Design review of the part built by this model. Coordinates are the model's own, in mm. A direction names the side the tool comes from. Coordinates: 2 decimals unless noted, no trailing zeros. Loops run counter-clockwise (first coordinate to the right, second up) from the corner with the lowest first, then second, coordinate; pieces in that order, holes last. Notation, with made-up numbers: (-2.75, -34.75) -> (17.25, -34.75) arc R9 ccw to (17.25, -18.75) -> close; hole circle Ø8 at (55.5, 66.25). An arc over 180 degrees is marked (long way). Use a Markdown table: item, result. Add a question column.
Q1. For faces 4 (the face through (-14.287, 14.248, 2.028)), 5 (the face through (11, -8, 11)), list the 3-axis set-ups (+Z, -Z, +X, -X, +Y, -Y) from which the entire face can be reached by the end or side of a thin tool; tool diameter is ignored.
Q2. For probe 1 along Y at (x, z) = (0, 1.2); probe 2 along X at (y, z) = (-5.5, 5); probe 3 along Z at (x, y) = (-6, 1.5), list the stretches that pass through material, from the lowest coordinate up.
Q3. Clearance check with flat-ended pins moving along their axes: pin 1 Ø6 at (x, y) = (-4, 0.5) entering from -Z; pin 2 Ø6 at (x, y) = (6, 6) entering from +Z; pin 3 Ø7.5 at (x, y) = (0, 0) entering from +Z. State where each tip first meets the part, or that it passes through.
Q4. Take a section at A-A on z = 29. Write out the cut boundary in (x, y), plus the area to 3 significant figures.
Q5. Draft analysis for pull direction X (two halves, no side actions). For faces 1 (the face through (0, 15, 2)), 2 (the face through (-15, -5, 12)), 3 (the face through (-11, -8, 11)), state which applies: pulls with the +X half, pulls with the -X half, needs draft (parallel to the pull), parting line crosses it, or undercut.
Q6. Take a section at D-D on y = -9. Write out the cut boundary in (x, z), plus the area to 3 significant figures.
Q7. Take a section at C-C on x = 0. Write out the cut boundary in (y, z), plus the area to 3 significant figures.
Q8. Take a section at B-B on y = 0. Write out the cut boundary in (x, z), plus the area to 3 significant figures.
from build123d import *

# Parameters (mm, degrees)
ESQUISSE1_W             = 30
ESQUISSE1_H             = 33
ESQUISSE1_R             = 4.25
BOSS_EXTRU_1_DEPTH      = 4
CONG_1_R                = 2.5
BOSS_EXTRU_2_DEPTH      = 4
BOSS_EXTRU_3_DEPTH      = 4
ESQUISSE5_R             = 150
ENL_V_MAT_EXTRU_1_DEPTH = 42.291645644


with BuildPart() as part:
    # Esquisse1 → Boss.-Extru.1 (new body)
    with BuildSketch(Plane.XY):
        with Locations((0, -1.5)):
            Rectangle(ESQUISSE1_W, ESQUISSE1_H)
        Circle(ESQUISSE1_R, mode=Mode.SUBTRACT)
    extrude(amount=BOSS_EXTRU_1_DEPTH)

    # Congé1
    cong_1_edges = [part.edges().sort_by_distance(p)[0] for p in [
        (-15, 15, 2),
        (15, 15, 2),
    ]]
    fillet(cong_1_edges, radius=CONG_1_R)

    # Esquisse2 → Boss.-Extru.2 (add)
    with BuildSketch(Plane(origin=(15, 0, 0), x_dir=(0, 0, -1), z_dir=(1, 0, 0))):
        Polygon((-4, -18), (-34, -18), (-4, 12), align=None)
    extrude(amount=-BOSS_EXTRU_2_DEPTH)

    # Esquisse4 → Boss.-Extru.3 (add)
    with BuildSketch(Plane.ZY.offset(15)):
        Polygon((4, -18), (34, -18), (4, 12), align=None)
    extrude(amount=-BOSS_EXTRU_3_DEPTH)

    # Esquisse5 → Enlèv. mat.-Extru.1 (cut, through all)
    with BuildSketch(Plane(origin=(0, 0, 0), x_dir=(-1, 0, 0), z_dir=(0, 0, -1))):
        with Locations((0, -165)):
            Circle(ESQUISSE5_R)
    extrude(amount=-ENL_V_MAT_EXTRU_1_DEPTH, mode=Mode.SUBTRACT)


solid = part.part
Answer list:
| question | item | result |
|---|---|---|
| 1 | face 4 | +Z, -Z, -X, +Y |
| 1 | face 5 | +Z, +Y, -Y |
| 2 | probe 1 | -15 to -4.25, 4.25 to 15 |
| 2 | probe 2 | -15 to -11, 11 to 15 |
| 2 | probe 3 | 0 to 4 |
| 3 | pin 1 | z = 0 |
| 3 | pin 2 | z = 4 |
| 3 | pin 3 | through |
| 4 | outline | (-15, -15.75) arc R150 cw to (-11, -15.4) -> (-11, -13) -> (-15, -13) -> close; (11, -15.4) arc R150 cw to (15, -15.75) -> (15, -13) -> (11, -13) -> close |
| 4 | area | 20.6 mm² |
| 5 | face 1 | needs draft |
| 5 | face 2 | pulls with the -X half |
| 5 | face 3 | undercut |
| 6 | outline | (-15, 0) -> (15, 0) -> (15, 25) -> (11, 25) -> (11, 4) -> (-11, 4) -> (-11, 25) -> (-15, 25) -> close |
| 6 | area | 288 mm² |
| 7 | outline | (-15, 0) -> (-4.25, 0) -> (-4.25, 4) -> (-15, 4) -> close; (4.25, 0) -> (15, 0) -> (15, 4) -> (4.25, 4) -> close |
| 7 | area | 86.0 mm² |
| 8 | outline | (-15, 0) -> (-4.25, 0) -> (-4.25, 4) -> (-11, 4) -> (-11, 16) -> (-15, 16) -> close; (4.25, 0) -> (15, 0) -> (15, 16) -> (11, 16) -> (11, 4) -> (4.25, 4) -> close |
| 8 | area | 182 mm² |
